The figure shows three views and two pictorial views of one solid part (mm, origin at its lowest corner). Answer the questions. Give positions to 0.01 mm unless a question says otherwise; leave off trailing zeros. Loops run counter-clockwise (first coordinate to the right, second up) from the corner with the lowest first, then second, coordinate; pieces in that order, holes last. Notation, with made-up numbers: M 2.5,-26.5 L 54.5,-26.5 A21 ccw 54.5,-20.5 Z; hole C 11.25,-17 d1. An arc over 180 degrees is marked long. One line per item, written item: value. Start each with the question number.
Q1. A cutting plane is placed at A-A, the plane x = 14.5. Determine the outline of the cut face in (y, z).
Q2. A cutting plane is placed at B-B, the plane z = 4.5. Determine the outline of the cut face in (x, y).
Q3. A flat-ended cylindrical pin translates along its axis: pin 1 (10 mm diameter, centred on x = 30, y = 62, fed in from -Z). Find the tip coordinate at first contact, or state that the pin passes through.
Q4. Consider L1, parallel to Z at x = 21.5, y = 55.5; L2, parallel to Z at x = 29.5, y = 50; L3, parallel to Y at x = 11.5, z = 5.25. Determine where each line is inside the solid, lowest interval first.
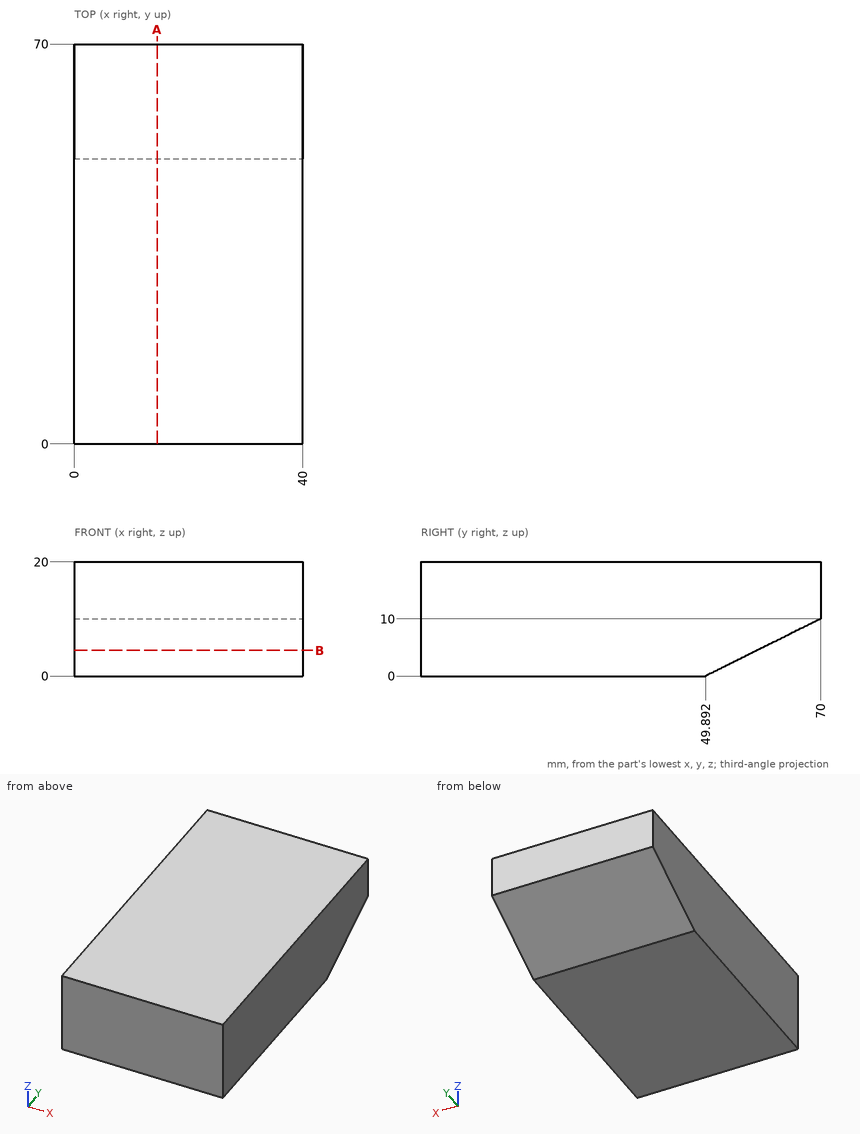
Answer block:
1. outline: M 0,0 L 49.89,0 L 70,10 L 70,20 L 0,20 Z
2. outline: M 0,0 L 40,0 L 40,58.94 L 0,58.94 Z
3. pin 1: z = 3.53
4. L1: 2.79 to 20
4. L2: 0.05 to 20
4. L3: 0 to 60.45
